For this review, take the finished solid that the model builds, in its own axes (mm). A direction names the side the tool comes from. Give positions to 0.01 mm unless a question says otherwise; leave off trailing zeros. Write each loop counter-clockwise with the first axis right and the second up, starting at its lowest first coordinate (ties: lowest second). Pieces come first, ordered by that corner, then holes.
from build123d import *

# Parameters (mm, degrees)
F0_R     = 10
F1_DEPTH = 10
F2_R     = 3.5
F3_DEPTH = 13.386621823


with BuildPart() as f1:
    # F0 (on Top) → F1 (new body)
    with BuildSketch(Plane.XY):
        with BuildLine():
            ThreePointArc((9, -9.3808315196), (11.9582607431, -5.0990195136), (13, 0))
            ThreePointArc((13, 0), (-5.0990195136, 11.9582607431), (-9, -9.3808315196))
            ThreePointArc((-9, -9.3808315196), (0, -13), (9, -9.3808315196))
        make_face()
        Circle(F0_R, mode=Mode.SUBTRACT)
        with BuildLine():
            ThreePointArc((9, -9.3808315196), (0, -13), (-9, -9.3808315196))
            Line((-9, -9.3808315196), (-9, -20))
            Line((-9, -20), (9, -20))
            Line((9, -20), (9, -9.3808315196))
        make_face()
    extrude(amount=F1_DEPTH)

    # F2 (on face) → F3 (cut, through all)
    with BuildSketch(Plane.XZ.offset(20)):
        with Locations((-4, 4.9318415113)):
            Circle(F2_R)
        with Locations((4, 4.9318415113)):
            Circle(F2_R)
    extrude(amount=-F3_DEPTH, mode=Mode.SUBTRACT)


solid = f1.part
(1) We need section B-B (y = -4). Write out the cut boundary in (x, z).
(2) Tool access review of faces 4 (the flat face through (0, -11, 10)), 5 (the cylindrical face through (-6.777, -14.888, 2.802)), 6 (the flat face through (9, -15, 5)): name each direction out of +Z, -Z, +X, -X, +Y, -Y from which nothing blocks a thin tool from reaching the whole face with its end or side.
(3) Clearance check with flat-ended pins moving along their axes: pin 1 Ø5 at (y, z) = (-16.5, 3.5) entering from +X; pin 2 Ø4 at (x, z) = (4, 4.93) entering from +Y; pin 3 Ø12 at (x, y) = (10.5, -10) entering from -Z; pin 4 Ø1.5 at (y, z) = (-8, 5.5) entering from +X. State where each tip first meets the part, or that it passes through.
(4) For L1, parallel to X at y = -13, z = 5; L2, parallel to Z at x = 4, y = -14.25; L3, parallel to X at y = -10.5, z = 6.25, list the stretches that pass through material, from the lowest coordinate up.
(5) We need section C-C (z = 3.75). Write out the cut boundary in (x, y).
(6) The part is to be moulded in two halves that separate along X. For faces 1 (the flat face through (0, -11, 0)), 2 (the cylindrical face through (7.233, -14.888, 3.591)), 3 (the flat face through (-9, -15, 5)), say which applies: +X half, -X half, draft (parallel to the pull), parting line (faces both ways), or undercut.
(7) We need section D-D (x = 4). Write out the cut boundary in (y, z), and give its area (3 significant figures).
(8) We need section A-A (x = 0). Write out the cut boundary in (y, z), and give its area (3 significant figures).
The answers:
1. outline: (-12.37, 0) - (-9.17, 0) - (-9.17, 10) - (-12.37, 10) - close; (9.17, 0) - (12.37, 0) - (12.37, 10) - (9.17, 10) - close
2. face 4: +Z, +X, -X, +Y, -Y
2. face 5: -Y
2. face 6: +Z, -Z, +X, -Y
3. pin 1: stops at x = 9
3. pin 2: stops at y = 12.85
3. pin 3: stops at z = 0
3. pin 4: stops at x = 10.79
4. L1: x = -9 to -7.5, -0.5 to 0.5, 7.5 to 9
4. L2: z = 0 to 1.43, 8.43 to 10
4. L3: x = -9 to -7.24, -0.76 to 0.76, 7.24 to 9
5. outline: (-9, -20) - (-7.29, -20) - (-7.29, -6.84) arc R10 cw (long way) to (7.29, -6.84) - (7.29, -20) - (9, -20) - (9, -9.38) arc R13 ccw (long way) to (-9, -9.38) - close; (-0.71, -20) - (0.71, -20) - (0.71, -9.98) arc R10 cw to (-0.71, -9.98) - close
6. face 1: draft
6. face 2: undercut
6. face 3: -X half
7. outline: (-20, 0) - (-9.17, 0) - (-9.17, 1.43) - (-20, 1.43) - close; (-20, 8.43) - (-9.17, 8.43) - (-9.17, 10) - (-20, 10) - close; (9.17, 0) - (12.37, 0) - (12.37, 10) - (9.17, 10) - close
7. area: 64.5 mm2
8. outline: (-20, 0) - (-10, 0) - (-10, 10) - (-20, 10) - close; (10, 0) - (13, 0) - (13, 10) - (10, 10) - close
8. area: 130 mm2
